Autodesk Inventor part; units mm, degrees
ref_plane "YZ Plane" through (0, 0, 0) normal (1, 0, 0) x (0, 1, 0)
ref_plane "XZ Plane" through (0, 0, 0) normal (0, 1, 0) x (-1, 0, 0)
ref_plane "XY Plane" through (0, 0, 0) normal (0, 0, 1) x (1, 0, 0)
sketch "Sketch1" plane through (0, 0, 0) normal (0, 0, 1) x (1, 0, 0)
  line L0 (-21, 20) -> (-21, -20) construction
  line L1 (14.2964, 21) -> (-14.2964, 21) construction
  line L2 (21, -20) -> (21, 20) construction
  line L3 (-14.2964, -21) -> (14.2964, -21) construction
  circle A0 centre (-14.3744, 12.3744) radius 1.621 construction
  circle A1 centre (10.3746, 12.3744) radius 1.621 construction
  circle A2 centre (10.3746, -12.3746) radius 1.621 construction
  circle A3 centre (-14.3744, -12.3746) radius 1.621 construction
  line L4 (-21, 21) -> (21, 21)
  line L5 (21, 21) -> (21, -21)
  line L6 (21, -21) -> (-21, -21)
  line L7 (-21, -21) -> (-21, 21)
  circle A4 centre (-14.3744, 12.3744) radius 2.1
  circle A5 centre (10.3746, 12.3744) radius 2.1
  circle A6 centre (10.3746, -12.3746) radius 2.1
  circle A7 centre (-14.3744, -12.3746) radius 2.1
  circle A8 centre (-2, 0) radius 11 construction
  circle A9 centre (-2, 0) radius 12
  point P0 (0, 0)
  dimension "d0" = 4.2
  dimension "d1" = 1
extrude "Extrusion1" add sketch "Sketch1" along normal blind 5
sketch "Sketch2" plane through (0, 0, 5) normal (0, 0, 1) x (1, 0, 0)
  line L0 (-21, -21) -> (21, -21)
  line L1 (21, 21) -> (-21, 21)
  line L2 (-21, 21) -> (-21, -21)
  line L3 (21, -21) -> (21, -25)
  line L4 (21, -25) -> (-25, -25)
  line L5 (-25, -25) -> (-25, 25)
  line L6 (-25, 25) -> (21, 25)
  line L7 (21, 25) -> (21, 21)
  point P0 (0, 0)
  dimension "d4" = 4
  dimension "d5" = 4
  dimension "d6" = 4
extrude "Extrusion2" add sketch "Sketch2" against normal blind 10
fillet "Fillet1" radius 4 2 edges at (-25, -25, 0) (-25, 25, 0)
properties part number "ShoulderEncoderDrillGuide"
The model under review builds one solid part; all positions refer to its coordinate system, in mm. A direction names the side the tool comes from. Give positions to 0.01 mm unless a question says otherwise; leave off trailing zeros. Write each loop counter-clockwise with the first axis right and the second up, starting at its lowest first coordinate (ties: lowest second). Pieces come first, ordered by that corner, then holes. Notation, with made-up numbers: (-31, 69) - (19, 69) arc R31 cw to (19, 95) - close; hole circle Ø7 at (19.5, 81.25). An arc over 180 degrees is marked (long way). Answer in a Markdown table with one row per item. Add a question column.
1. Draft analysis for pull direction X (two halves, no side actions). For faces 1 (the cylindrical face through (-12.435, -11.57, 2.465)), 2 (the cylindrical face through (-23.797, -23.859, -0.07)), 3 (the flat face through (-21, 0, -2)), 4 (the flat face through (9, 10, 0)), state which applies: +X half, -X half, draft (parallel to the pull), parting line (faces both ways), or undercut.
2. We need section A-A on y = 0. Write out the cut boundary in (x, z), then the cut area to 3 significant figures.
3. We need section B-B on x = -2. Write out the cut boundary in (y, z), then the cut area to 3 significant figures.
4. We need section C-C on z = -3.5. Write out the cut boundary in (x, y).
5. We need section D-D on x = -17.5. Write out the cut boundary in (y, z).
6. Wall thickness on line 1 along Y through (x, z) = (13.5, -3.75); line 2 along Z through (x, y) = (-1, -14.5); line 3 along X through (y, z) = (-3, -1): over which ranges is each line inside the solid? List them lowest first. Write a range as [from, to].
7. Insertion check: P1, Ø1, axis at y = -7.5, z = -2, coming from the +X side; P2, Ø3.5, axis at x = -14.37, y = 12.37, coming from the +Z side (3 decimals); P3, Ø6.5, axis at x = 10.37, y = 12.37, coming from the -Z side. Each pin has a flat end and moves straight along its axis. Give the tip position at first contact, or say it passes through.
8. Tool access review of faces 5 (the cylindrical face through (-11.523, 7.302, 2.465)), 6 (the flat face through (0, -21, -2)): name each direction out of +Z, -Z, +X, -X, +Y, -Y from which nothing blocks a thin tool from reaching the whole face with its end or side.
Ans:
| question | item | result |
|---|---|---|
| 1 | face 1 | undercut |
| 1 | face 2 | -X half |
| 1 | face 3 | +X half |
| 1 | face 4 | draft |
| 2 | outline | (-25, -5) - (-21, -5) - (-21, 0) - (-14, 0) - (-14, 5) - (-25, 5) - close; (10, 0) - (21, 0) - (21, 5) - (10, 5) - close |
| 2 | area | 130 mm^2 |
| 3 | outline | (-25, -5) - (-21, -5) - (-21, 0) - (-12, 0) - (-12, 5) - (-25, 5) - close; (12, 0) - (21, 0) - (21, -5) - (25, -5) - (25, 5) - (12, 5) - close |
| 3 | area | 170 mm^2 |
| 4 | outline | (-25, -21) arc R4 ccw to (-21, -25) - (21, -25) - (21, -21) - (-21, -21) - (-21, 21) - (21, 21) - (21, 25) - (-21, 25) arc R4 ccw to (-25, 21) - close |
| 5 | outline | (-25, -5) - (-21, -5) - (-21, 0) - (21, 0) - (21, -5) - (25, -5) - (25, 5) - (-25, 5) - close |
| 6 | line 1 | y = [-25, -21], [21, 25] |
| 6 | line 2 | z = [0, 5] |
| 6 | line 3 | x = [-25, -21] |
| 7 | P1 | stops at x = -21 |
| 7 | P2 | passes through |
| 7 | P3 | stops at z = 0 |
| 8 | face 5 | +Z, -Z |
| 8 | face 6 | -Z, +X |
